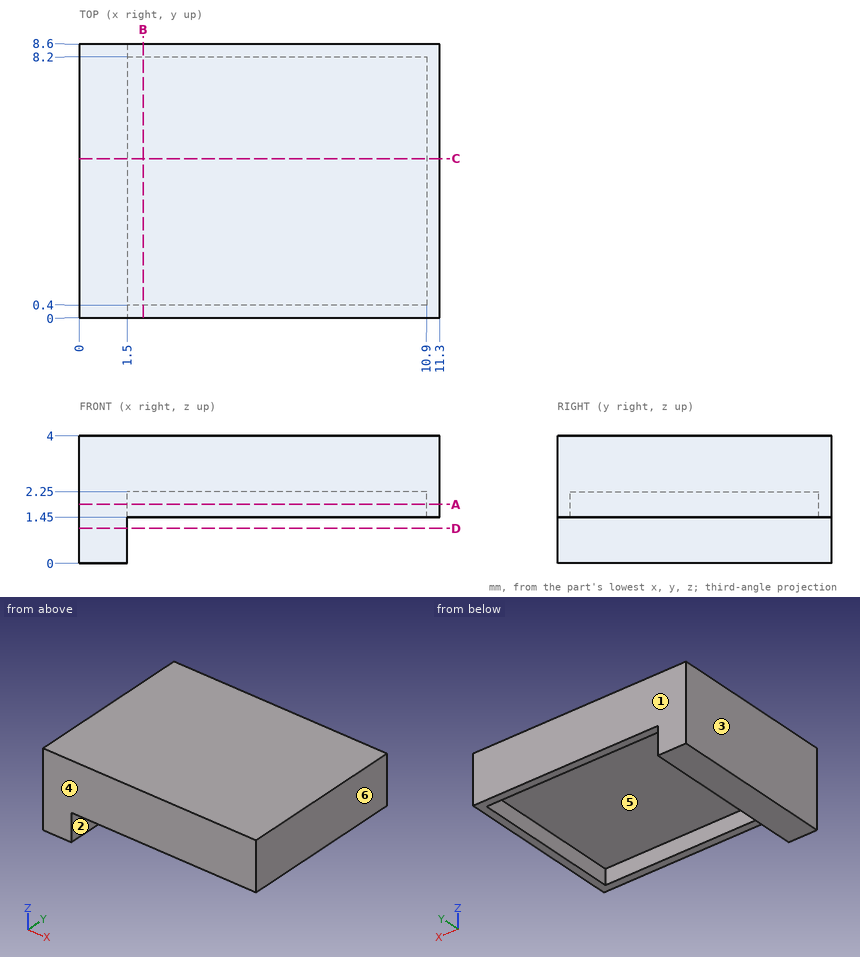
Source: three-view drawing plus pictorial views. Frame: mm from the lowest corner of the part. A direction names the side the tool comes from. Coordinates: 2 decimals unless noted, no trailing zeros. Order: outer loops, then holes, each group sorted by start corner. A loop starts at its lowest first (then second) coordinate and runs counter-clockwise, first axis right, second up.
1) Set-up query: the marked faces 1 and 2. Return all of +Z, -Z, +X, -X, +Y, -Y with unobstructed straight access to the full face (end or side cutting, diameter ignored); none if empty.
Result sheet:
face 1: +Z, -Z, +X, -X, +Y
face 2: -Z
2) Section A-A (z = 1.85). Return loops of the section in (x, y), then the cut area to 3 significant figures.
Result sheet:
outline: (0, 0) - (11.3, 0) - (11.3, 8.6) - (0, 8.6) - close; hole (1.5, 0.4) - (10.9, 0.4) - (10.9, 8.2) - (1.5, 8.2) - close
area: 23.9 mm2
3) Section D-D (z = 1.1). Return loops of the section in (x, y), then the cut area to 3 significant figures.
Result sheet:
outline: (0, 0) - (1.5, 0) - (1.5, 8.6) - (0, 8.6) - close
area: 12.9 mm2
4) Draft query along X for the marked faces 3, 4, 5 and 6. Return one class per face: released by +X, released by -X, zero draft, split by the parting line, or undercut.
Result sheet:
face 3: released by -X
face 4: zero draft
face 5: undercut
face 6: released by +X
5) First-contact query: P1, Ø2.5, axis at x = 8, y = 5, coming from the -Z side. Flat tip, straight axial feed; report the tip coordinate or a pass-through.
Result sheet:
P1: stops at z = 2.25
6) Section C-C (y = 5). Return loops of the section in (x, z).
Result sheet:
outline: (0, 0) - (1.5, 0) - (1.5, 2.25) - (10.9, 2.25) - (10.9, 1.45) - (11.3, 1.45) - (11.3, 4) - (0, 4) - close
7) Ray query, probe 1 along X at (y, z) = (2.25, 1.55); probe 2 along Y at (x, z) = (4.5, 1.5); probe 3 along X at (y, z) = (4.25, 1.1). Return the intervals inside material, ascending.
Result sheet:
probe 1: x = 0 to 1.5, 10.9 to 11.3
probe 2: y = 0 to 0.4, 8.2 to 8.6
probe 3: x = 0 to 1.5
8) Section B-B (x = 2). Return loops of the section in (y, z).
Result sheet:
outline: (0, 1.45) - (0.4, 1.45) - (0.4, 2.25) - (8.2, 2.25) - (8.2, 1.45) - (8.6, 1.45) - (8.6, 4) - (0, 4) - close
